Check sheet for the modelled part. Datum: model origin and axes. Units: mm. Face numbers are marked on the shaded views. A direction names the side the tool comes from. Coordinates: 2 decimals unless noted, no trailing zeros. Loops run counter-clockwise (first coordinate to the right, second up) from the corner with the lowest first, then second, coordinate; pieces in that order, holes last. Notation, with made-up numbers: (18, 84.5) - (43, 84.5) arc R18 ccw to (43, 90.5) - close; hole circle Ø9 at (57.25, -39.5). An arc over 180 degrees is marked (long way). Use a Markdown table: item, result. Add a question column.
1) Thickness scan on line 1 (X direction, y = 2.2, z = -5.27) (3 decimals); line 2 (Z direction, x = -0.5, y = 0.75); line 3 (Y direction, x = -13, z = -26). Record the ranges inside material, lowest first.
2) Tool access check on the marked faces 1, 2 and 3. Record the directions out of +Z, -Z, +X, -X, +Y, -Y that give a thin tool (end or side, any length) a straight path to the whole face; none if there is none.
3) Go/stop test with flat-tipped pins: P1, Ø10, axis at x = -5, y = -6.5, coming from the +Z side; P2, Ø1.5, axis at x = 4.5, z = 1, coming from the -Y side; P3, Ø3.5, axis at y = -1.82, z = -28.3, coming from the +X side; P4, Ø5, axis at x = -0.5, y = -4, coming from the -Z side. Record where each tip stops, or that it passes through.
4) Sectioned sample at A-A, the plane x = 0. Enter the section's corners in (y, z), then the cut area to 3 significant figures.
5) Sectioned sample at D-D, the plane x = -12. State how many separate pieces and enclosed holes the cut face has, then the cut area to 3 significant figures.
6) Draft check along X on the marked faces 4, 5 and 6. Enter one of: pulls with the +X half, pulls with the -X half, needs draft (parallel to the pull), parting line crosses it, or undercut.
7) Sectioned sample at B-B, the plane z = 5. Enter the section's corners in (x, y), then the cut area to 3 significant figures.
8) Sectioned sample at C-C, the plane x = -5. Enter the section's corners in (y, z), then the cut area to 3 significant figures.
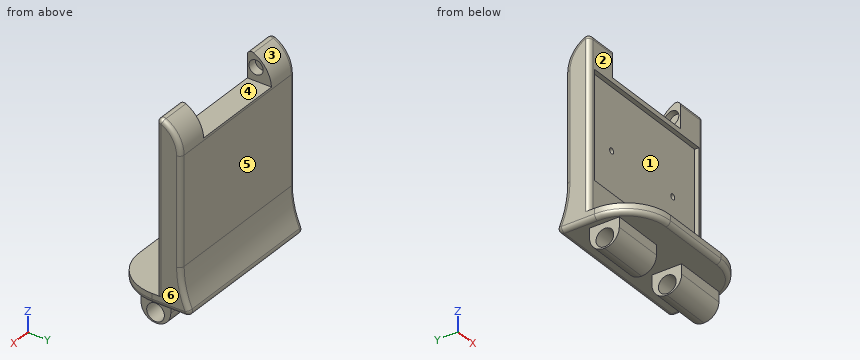
from build123d import *

# Parameters (mm, degrees)
BOSS_EXTRUDE1_DEPTH     = 18
SKETCH2_W               = 21.5
SKETCH2_H               = 6.5
CUT_EXTRUDE1_DEPTH      = 36
FILLET1_R               = 1
FILLET2_R               = 10
SKETCH3_R               = 1.6
CUT_EXTRUDE2_DEPTH      = 23
CUT_EXTRUDE2_DEPTH_BACK = 2
SKETCH4_W               = 11.8
SKETCH4_H               = 6.7
BOSS_EXTRUDE2_DEPTH     = 5.6
CUT_EXTRUDE3_DEPTH      = 34.8
SKETCH6_R               = 2
CUT_EXTRUDE4_DEPTH      = 34.8
SKETCH7_W               = 33.22
SKETCH7_H               = 24.2
CUT_EXTRUDE5_DEPTH      = 1
M1_6_TAPPED_HOLE1_D     = 1.25
M1_6_TAPPED_HOLE1_DEPTH = 3
M1_6_TAPPED_HOLE1_TIP   = 0.375537887
FILLET3_R               = 1
FILLET4_R               = 1


with BuildPart() as part:
    # Sketch1 → Boss-Extrude1 (new body, symmetric)
    with BuildSketch(Plane(origin=(0, 0, 0), x_dir=(0, 0, -1), z_dir=(1, 0, 0))):
        with BuildLine():
            Line((-16.23, 0), (22.77, 0))
            Line((22.77, 0), (22.77, -11.06))
            Line((22.77, -11.06), (25, -11.06))
            Line((25, -11.06), (25, 8.04))
            ThreePointArc((25, 8.04), (20.158769233, 6.144924279), (15, 5.5))
            Line((15, 5.5), (-9.23, 5.5))
            ThreePointArc((-9.23, 5.5), (-13.681123454, 3.960520759), (-16.23, 0))
        make_face()
    extrude(amount=BOSS_EXTRUDE1_DEPTH, both=True)

    # Sketch2 → Cut-Extrude1 (cut)
    with BuildSketch(Plane(origin=(0, 5.5, 0), x_dir=(1, 0, 0), z_dir=(0, 1, 0))):
        with Locations((0, -12.98)):
            Rectangle(SKETCH2_W, SKETCH2_H)
    extrude(amount=-CUT_EXTRUDE1_DEPTH, mode=Mode.SUBTRACT)

    # Fillet1
    fillet1_edges = [part.edges().sort_by_distance(p)[0] for p in [
        (0, 8.04, -25),
    ]]
    fillet(fillet1_edges, radius=FILLET1_R)

    # Fillet2
    fillet2_edges = [part.edges().sort_by_distance(p)[0] for p in [
        (18, -11.06, -23.885),
        (-18, -11.06, -23.885),
    ]]
    fillet(fillet2_edges, radius=FILLET2_R)

    # Sketch3 → Cut-Extrude2 (cut, two sides)
    with BuildSketch(Plane(origin=(-10.75, 0, 0), x_dir=(0, 0, -1), z_dir=(1, 0, 0))) as cut_extrude2_sk:
        with Locations((-12.73, 1.9826289)):
            Circle(SKETCH3_R)
    extrude(amount=CUT_EXTRUDE2_DEPTH, mode=Mode.SUBTRACT)
    extrude(cut_extrude2_sk.sketch, amount=-CUT_EXTRUDE2_DEPTH_BACK, mode=Mode.SUBTRACT)

    # Sketch4 → Boss-Extrude2 (add)
    with BuildSketch(Plane(origin=(0, 0, -25), x_dir=(-1, 0, 0), z_dir=(0, 0, -1))):
        with Locations((-9.9, -1.720538118)):
            Rectangle(SKETCH4_W, SKETCH4_H)
        with Locations((9.9, -1.720538118)):
            Rectangle(SKETCH4_W, SKETCH4_H)
    extrude(amount=BOSS_EXTRUDE2_DEPTH)

    # Sketch5 → Cut-Extrude3 (cut, through all)
    with BuildSketch(Plane(origin=(15.8, 0, 0), x_dir=(0, 0, -1), z_dir=(1, 0, 0))):
        with BuildLine():
            Line((30.6, -1.720538118), (30.6, 1.629461882))
            Line((30.6, 1.629461882), (27.25, 1.629461882))
            ThreePointArc((27.25, 1.629461882), (29.618807717, 0.648269599), (30.6, -1.720538118))
        make_face()
        with BuildLine():
            Line((30.6, -5.070538118), (30.6, -1.720538118))
            ThreePointArc((30.6, -1.720538118), (29.618807717, -4.089345835), (27.25, -5.070538118))
            Line((27.25, -5.070538118), (30.6, -5.070538118))
        make_face()
    extrude(amount=-CUT_EXTRUDE3_DEPTH, mode=Mode.SUBTRACT)

    # Sketch6 → Cut-Extrude4 (cut, through all)
    with BuildSketch(Plane(origin=(15.8, 0, 0), x_dir=(0, 0, -1), z_dir=(1, 0, 0))):
        with Locations((28.302174941, -1.820538118)):
            Circle(SKETCH6_R)
    extrude(amount=-CUT_EXTRUDE4_DEPTH, mode=Mode.SUBTRACT)

    # Sketch7 → Cut-Extrude5 (cut)
    with BuildSketch(Plane.XZ):
        with Locations((0, -3.47)):
            Rectangle(SKETCH7_W, SKETCH7_H)
    extrude(amount=-CUT_EXTRUDE5_DEPTH, mode=Mode.SUBTRACT)

    # M1.6 Tapped Hole1
    with Locations(Plane(origin=(0, 1, 0), x_dir=(-1, 0, 0), z_dir=(0, -1, 0))):
        with Locations((9.7, 5.27), (-9.7, 5.27)):
            Hole(M1_6_TAPPED_HOLE1_D / 2, depth=M1_6_TAPPED_HOLE1_DEPTH)
            with Locations((0, 0, -(M1_6_TAPPED_HOLE1_DEPTH + M1_6_TAPPED_HOLE1_TIP / 2))):  # 118° drill point
                Cone(0, M1_6_TAPPED_HOLE1_D / 2, M1_6_TAPPED_HOLE1_TIP, mode=Mode.SUBTRACT)

    # Fillet3
    fillet3_edges = [part.edges().sort_by_distance(p)[0] for p in [
        (14.375, 0, 16.23),
        (-14.375, 0, 16.23),
    ]]
    fillet(fillet3_edges, radius=FILLET3_R)

    # Fillet4
    fillet4_edges = [part.edges().sort_by_distance(p)[0] for p in [
        (-18, 0, -3.977965877),
        (18, 0, -3.977965877),
        (-18, 0.468914995, 15.661386792),
        (18, 0.468914995, 15.661386792),
        (18, 5.5, -2.885),
        (18, 4.399999523, 13.056226055),
        (-18, 5.96556671, -19.392628497),
        (18, 5.96556671, -19.392628497),
        (-18, 7.269083423, -24.543171858),
        (18, 7.269083423, -24.543171858),
        (0, -11.06, -25),
        (-18, 2.684730941, -25),
        (18, 2.684730941, -25),
        (15.071067812, -8.131067812, -25),
        (-15.071067812, -8.131067812, -25),
        (-18, 5.5, -2.885),
        (-18, 4.399999523, 13.056226055),
    ]]
    fillet(fillet4_edges, radius=FILLET4_R)


solid = part.part
Solved:
| question | item | result |
|---|---|---|
| 1 | line 1 | x = -18 to -10.325, -9.075 to 9.075, 10.325 to 18 |
| 1 | line 2 | z = -25 to -15.57, 8.63 to 9.73 |
| 1 | line 3 | y = -5.07 to 1.63 |
| 2 | face 1 | -Y |
| 2 | face 2 | +Z, +X, -X, -Y |
| 2 | face 3 | +Z, +X, -X, +Y |
| 3 | P1 | stops at z = -22.77 |
| 3 | P2 | stops at y = 1 |
| 3 | P3 | passes through |
| 3 | P4 | stops at z = -25 |
| 4 | outline | (-11.06, -24) arc R1 ccw to (-10.06, -25) - (6.43, -25) arc R1 ccw to (7.34, -23.59) arc R20.96 cw to (5.5, -15) - (5.5, 9.23) arc R7.2 ccw to (5.48, 9.73) - (0, 9.73) - (0, 8.63) - (1, 8.63) - (1, -15.57) - (0, -15.57) - (0, -22.77) - (-11.06, -22.77) - close |
| 4 | area | 199 mm2 |
| 5 | separate pieces | 1 |
| 5 | enclosed holes | 2 |
| 5 | area | 235 mm2 |
| 6 | face 4 | undercut |
| 6 | face 5 | needs draft |
| 6 | face 6 | pulls with the +X half |
| 7 | outline | (-18, 1) arc R1 ccw to (-17, 0) - (-16.61, 0) - (-16.61, 1) - (16.61, 1) - (16.61, 0) - (17, 0) arc R1 ccw to (18, 1) - (18, 4.5) arc R1 ccw to (17, 5.5) - (-17, 5.5) arc R1 ccw to (-18, 4.5) - close |
| 7 | area | 164 mm2 |
| 8 | outline | (-11.06, -24) arc R1 ccw to (-10.06, -25) - (-5.07, -25) - (-5.07, -27.25) arc R3.35 ccw to (1.63, -27.25) - (1.63, -25) - (6.43, -25) arc R1 ccw to (7.34, -23.59) arc R20.96 cw to (5.5, -15) - (5.5, 9.23) arc R7.2 ccw to (5.48, 9.73) - (0, 9.73) - (0, 8.63) - (1, 8.63) - (1, -15.57) - (0, -15.57) - (0, -22.77) - (-11.06, -22.77) - close; hole circle Ø4 at (-1.82, -28.3) |
| 8 | area | 219 mm2 |
